Can you work these out from the model? Positions are in its coordinate system, mm. Face numbers are marked on the shaded views. A direction names the side the tool comes from. Coordinates: 2 decimals unless noted, no trailing zeros. Loops run counter-clockwise (first coordinate to the right, second up) from the corner with the lowest first, then second, coordinate; pieces in that order, holes last.
```python
from build123d import *

# Parameters (mm, degrees)
SKETCH_1_R       = 2.7
SKETCH_1_R_2     = 2.2
EXTRUDE_1_DEPTH  = 5
SKETCH_1_4_W     = 29.647183795
SKETCH_1_4_H     = 2
EXTRUDE_2_DEPTH  = 6.8
CHAMFER_1_SIZE   = 3
CHAMFER_1_SIZE_2 = 6.8
CHAMFER_2_SIZE   = 3
CHAMFER_2_SIZE_2 = 6.8


with BuildPart() as part:
    # 草图1 → 凸台-拉伸1 (new body)
    with BuildSketch(Plane.XY):
        with BuildLine():
            Line((-22.414990858, 31.366560458), (-46.243327239, 8.911040306))
            ThreePointArc((-46.243327239, 8.911040306), (-47.17241807, 7.585353438), (-47.5, 6))
            Line((-47.5, 6), (-47.5, -6))
            ThreePointArc((-47.5, -6), (-47.17241807, -7.585353438), (-46.243327239, -8.911040306))
            Line((-46.243327239, -8.911040306), (-22.414990858, -31.366560458))
            ThreePointArc((-22.414990858, -31.366560458), (-19.606220239, -32.85608988), (-16.430695985, -32.701377246))
            Line((-16.430695985, -32.701377246), (20.169304015, -20.701377246))
            ThreePointArc((20.169304015, -20.701377246), (23.158797387, -18.520239758), (24.3, -15))
            Line((24.3, -15), (24.3, 15))
            ThreePointArc((24.3, 15), (23.158797387, 18.520239758), (20.169304015, 20.701377246))
            Line((20.169304015, 20.701377246), (-16.430695985, 32.701377246))
            ThreePointArc((-16.430695985, 32.701377246), (-19.606220239, 32.85608988), (-22.414990858, 31.366560458))
        make_face()
        with Locations((18.3, -15)):
            Circle(SKETCH_1_R, mode=Mode.SUBTRACT)
        with Locations((-38, 0)):
            Circle(SKETCH_1_R_2, mode=Mode.SUBTRACT)
        with Locations((-18, 0)):
            Circle(SKETCH_1_R_2, mode=Mode.SUBTRACT)
        with Locations((-18.3, 27)):
            Circle(SKETCH_1_R, mode=Mode.SUBTRACT)
        with Locations((18.3, 15)):
            Circle(SKETCH_1_R, mode=Mode.SUBTRACT)
        with Locations((-18.3, -27)):
            Circle(SKETCH_1_R, mode=Mode.SUBTRACT)
    extrude(amount=EXTRUDE_1_DEPTH)

    # 草图4 → 旋转1 (revolve)
    with BuildSketch(Plane(origin=(6.216937636, 18.961659791, 0), x_dir=(-0.9502295409734977, 0.31155066917163887, 0), z_dir=(-0.31155066917163887, -0.9502295409734977, 0)), mode=Mode.PRIVATE) as revolve_1_sk:
        Polygon((-6.715940562, 0), (-7.715940562, 7.7), (-10.015940562, 7.7), (-10.015940562, 0), align=None)
    revolve_1 = revolve(revolve_1_sk.sketch.rotate(Axis((18.3, 15, 4.45283877), (0, 0, -1)), 161.847294113), axis=Axis((18.3, 15, 4.45283877), (0, 0, -1)))

    # 草图4<3> → 旋转2 (revolve)
    with BuildSketch(Plane(origin=(6.216937636, 18.961659791, 0), x_dir=(-0.9502295409734977, 0.31155066917163887, 0), z_dir=(-0.31155066917163887, -0.9502295409734977, 0)), mode=Mode.PRIVATE) as revolve_2_sk:
        Polygon((30.801068667, 7.7), (28.501068667, 7.7), (28.501068667, 0), (31.801068667, 0), align=None)
    revolve_2 = revolve(revolve_2_sk.sketch.rotate(Axis((-18.3, 27, 0), (0, 0, -1)), 161.847294113), axis=Axis((-18.3, 27, 0), (0, 0, -1)))

    # 镜向1: 旋转1, 旋转2 across plane
    add(revolve_1.mirror(Plane.ZX))
    add(revolve_2.mirror(Plane.ZX))

    # 草图1<4> → 凸台-拉伸2 (add)
    with BuildSketch(Plane.XY):
        with Locations((-27.823591898, 11.3)):
            Rectangle(SKETCH_1_4_W, SKETCH_1_4_H)
        with Locations((-27.823591898, -11.3)):
            Rectangle(SKETCH_1_4_W, SKETCH_1_4_H)
    extrude(amount=-EXTRUDE_2_DEPTH)

    # 倒角1
    # the kernel refuses this chamfer: 6.8, 3 mm, written as the material it adds along each edge
    with BuildSketch(Plane(origin=(-13, 12.3, 0), x_dir=(0, 0.9968133817371192, 0.07976892872421078), z_dir=(-1, 0, 0))) as chamfer_1_piece_1_section:
        Polygon((CHAMFER_1_SIZE * 0.996813381737, CHAMFER_1_SIZE * 0.0797689287242), (-CHAMFER_1_SIZE_2 * 0.0797689287242, CHAMFER_1_SIZE_2 * 0.996813381737), (0, 0), align=None)
    chamfer_1_piece_1 = extrude(amount=29.647183795, mode=Mode.PRIVATE)
    chamfer_1_piece_1 = split(chamfer_1_piece_1, bisect_by=Plane(origin=(-34.073753533, 20.379491281, -2.31410284), z_dir=(0.685831809699718, -0.7277600764015637, 0)), keep=Keep.TOP, mode=Mode.PRIVATE)
    chamfer_1_piece_1 = split(chamfer_1_piece_1, bisect_by=Plane(origin=(-27.32988888, 13.223341061, -6.8), z_dir=(0, 0, 1)), keep=Keep.TOP, mode=Mode.PRIVATE)
    add(chamfer_1_piece_1)

    # 倒角2
    # the kernel refuses this chamfer: 6.8, 3 mm, written as the material it adds along each edge
    with BuildSketch(Plane(origin=(-42.647183795, -12.3, 0), x_dir=(0, -0.9968133817371192, 0.07976892872421078), z_dir=(1, 0, 0))) as chamfer_2_piece_1_section:
        Polygon((CHAMFER_2_SIZE * 0.996813381737, CHAMFER_2_SIZE * 0.0797689287242), (-CHAMFER_2_SIZE_2 * 0.0797689287242, CHAMFER_2_SIZE_2 * 0.996813381737), (0, 0), align=None)
    chamfer_2_piece_1 = extrude(amount=29.647183795, mode=Mode.PRIVATE)
    chamfer_2_piece_1 = split(chamfer_2_piece_1, bisect_by=Plane(origin=(-34.073753533, -20.379491281, -2.31410284), z_dir=(0.6858318096997175, 0.7277600764015641, 0)), keep=Keep.TOP, mode=Mode.PRIVATE)
    chamfer_2_piece_1 = split(chamfer_2_piece_1, bisect_by=Plane(origin=(-27.32988888, -13.223341061, -6.8), z_dir=(0, 0, 1)), keep=Keep.TOP, mode=Mode.PRIVATE)
    add(chamfer_2_piece_1)


solid = part.part
```
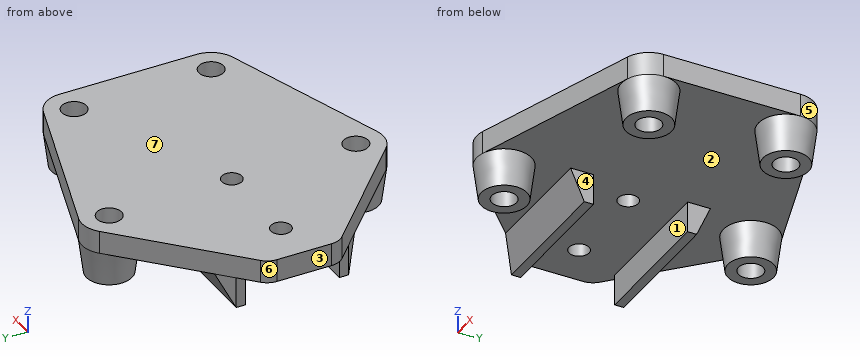
(1) I want a section at A-A on z = -3. State how many separate pieces and enclosed holes the cut face has, then the cut area to 3 significant figures.
Check values:
separate pieces: 6
enclosed holes: 4
area: 519 mm2
(2) Which directions (+Z, -Z, +X, -X, +Y, -Y) give clear straight access to the entire face, cutting with the end or side of a thin tool? Please do the marked faces 1, 2 and 3.
Check values:
face 1: -Z, -X
face 2: -Z
face 3: +Z, -Z, -X, +Y, -Y
(3) If I drill on probe 1 along Y at (x, z) = (-18, 2.05); probe 2 along Y at (x, z) = (18.3, -4.25); probe 3 along Y at (x, z) = (18.3, 1.7), over which ranges is the centre line in solid material (lowest first)?
Check values:
probe 1: y = -32.99 to -29.68, -24.32 to -2.2, 2.2 to 24.32, 29.68 to 32.99
probe 2: y = -20.45 to -17.7, -12.3 to -9.55, 9.55 to 12.3, 17.7 to 20.45
probe 3: y = -21.31 to -17.7, -12.3 to 12.3, 17.7 to 21.31
(4) I'm going to push flat-ended pins straight in: pin 1 (2.5 mm diameter, centred on y = -13, z = -3, fed in from +X); pin 2 (6 mm diameter, centred on x = -24, z = -5.5, fed in from +Y); pin 3 (1 mm diameter, centred on x = -24, y = -11.5, fed in from -Z). Where does each tip first touch, or does it pass through?
Check values:
pin 1: stops at x = 23.92
pin 2: stops at y = 31.6
pin 3: stops at z = -6.8
(5) I want a section at B-B on y = 0. Write out the boundary of the cut face in (x, z).
Check values:
outline: (-47.5, 0) - (-40.2, 0) - (-40.2, 5) - (-47.5, 5) - close; (-35.8, 0) - (-20.2, 0) - (-20.2, 5) - (-35.8, 5) - close; (-15.8, 0) - (24.3, 0) - (24.3, 5) - (-15.8, 5) - close
(6) I want a section at C-C on x = 18.3. Write out the boundary of the cut face in (y, z).
Check values:
outline: (-21.31, 0) - (-21, 0) - (-20, -7.7) - (-17.7, -7.7) - (-17.7, 5) - (-21.31, 5) - close; (-12.3, -7.7) - (-10, -7.7) - (-9, 0) - (9, 0) - (10, -7.7) - (12.3, -7.7) - (12.3, 5) - (-12.3, 5) - close; (17.7, -7.7) - (20, -7.7) - (21, 0) - (21.31, 0) - (21.31, 5) - (17.7, 5) - close
(7) If we mould it in two halves opening along X, with no side actions, what happens to the marked faces 4, 5, 6 and 7? For each: released by +X, released by -X, zero draft, split by the parting line, or undercut.
Check values:
face 4: undercut
face 5: released by +X
face 6: released by -X
face 7: zero draft
(8) I want a section at D-D on x = -38. Write out the boundary of the cut face in (y, z).
Check values:
outline: (-16.68, 0) - (-15.3, 0) - (-12.3, -6.8) - (-10.3, -6.8) - (-10.3, 0) - (-2.2, 0) - (-2.2, 5) - (-16.68, 5) - close; (2.2, 0) - (10.3, 0) - (10.3, -6.8) - (12.3, -6.8) - (15.3, 0) - (16.68, 0) - (16.68, 5) - (2.2, 5) - close
